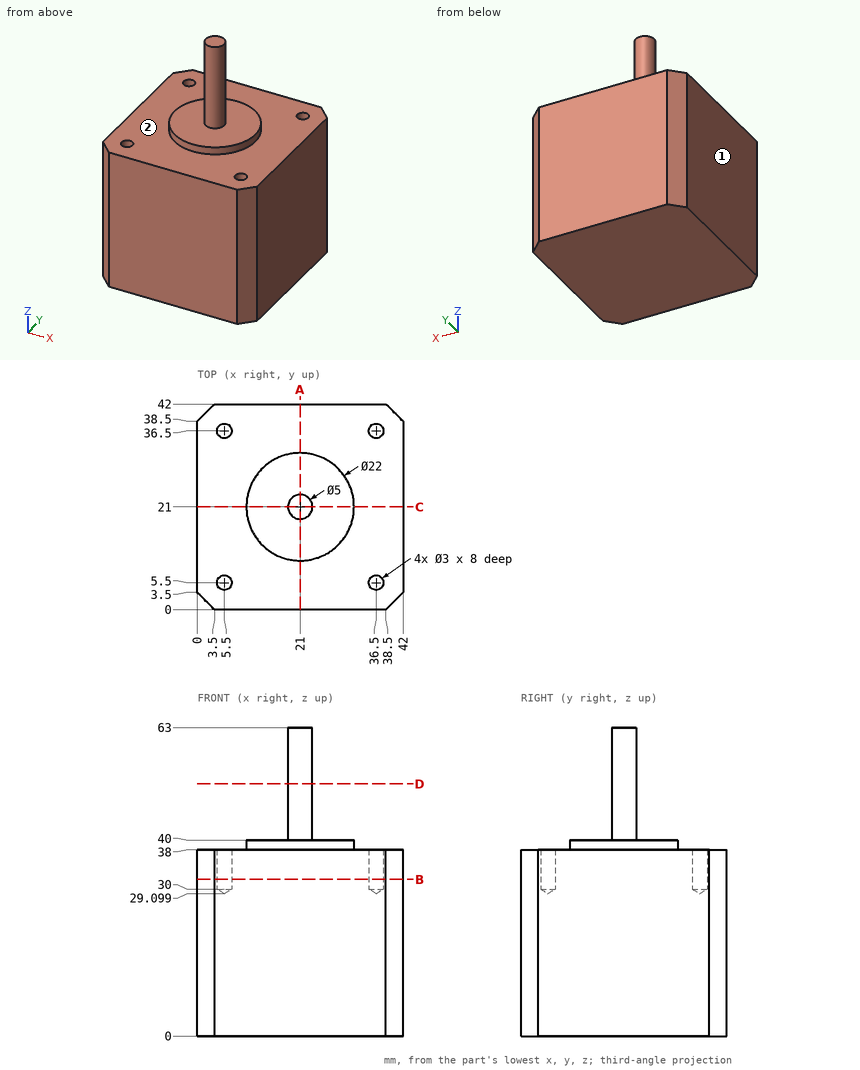
Design review of the part shown in the three views and the two pictorial views. Dimensions are in mm from the part's minimum x, y and z. A direction names the side the tool comes from. Round coordinates to 2 decimals unless told otherwise and drop trailing zeros. Write each loop counter-clockwise with the first axis right and the second up, starting at its lowest first coordinate (ties: lowest second). Pieces come first, ordered by that corner, then holes. Notation, with made-up numbers: (31, 39) - (67, 39) arc R24 cw to (67, 61) - close; hole circle Ø2 at (3.5, -20.75). An arc over 180 degrees is marked (long way). Return JSON: item names as keys, results as strings. Group by question number.
Item 1: We need section A-A on x = 21. Write out the cut boundary in (y, z).
Item 2: For probe 1 along Y at (x, z) = (5.5, 33.25); probe 2 along X at (y, z) = (5, 35) (1 decimal), list the stretches that pass through material, from the lowest coordinate up. Write a range as [from, to].
Item 3: We need section B-B on z = 32. Write out the cut boundary in (x, y), and give its area (3 significant figures).
Item 4: Machinability: for the marked faces 1 and 2, which of the approach directions +Z, -Z, +X, -X, +Y, -Y give a long, thin tool a straight path to every point of the face, cutting with its end or side? Answer none if there is none.
Item 5: We need section D-D on z = 51.5. Write out the cut boundary in (x, y).
Item 6: Insertion check: P1, Ø1, axis at x = 31, y = 30, coming from the +Z side; P2, Ø1.5, axis at x = 17, y = 24.5, coming from the +Z side; P3, Ø6, axis at x = 29.5, z = 42.5, coming from the -Y side (1 decimal). Each pin has a flat end and moves straight along its axis. Give the tip position at first contact, or say it passes through.
Model answer:
{
 "1": {"outline": "(0, 0) - (42, 0) - (42, 38) - (32, 38) - (32, 40) - (23.5, 40) - (23.5, 63) - (18.5, 63) - (18.5, 40) - (10, 40) - (10, 38) - (0, 38) - close"},
 "2": {"probe 1": "y = [0, 4], [7, 35], [38, 42]", "probe 2": "x = [0, 4.1], [6.9, 35.1], [37.9, 42]"},
 "3": {"outline": "(0, 3.5) - (3.5, 0) - (38.5, 0) - (42, 3.5) - (42, 38.5) - (38.5, 42) - (3.5, 42) - (0, 38.5) - close; hole circle Ø3 at (5.5, 5.5); hole circle Ø3 at (5.5, 36.5); hole circle Ø3 at (36.5, 5.5); hole circle Ø3 at (36.5, 36.5)", "area": "1,710 mm²"},
 "4": {"face 1": "+Z, -Z, -X, +Y, -Y", "face 2": "+Z"},
 "5": {"outline": "circle Ø5 at (21, 21)"},
 "6": {"P1": "stops at z = 38", "P2": "stops at z = 40", "P3": "stops at y = 12.4"}
}
